The model under review builds one solid part; all positions refer to its coordinate system, in mm. Face numbers are marked on the shaded views. Round coordinates to 2 decimals unless told otherwise and drop trailing zeros. Order: outer loops, then holes, each group sorted by start corner. A loop starts at its lowest first (then second) coordinate and runs counter-clockwise, first axis right, second up.
from build123d import *

# Parameters (mm, degrees)
SKETCH1_W           = 76.2
SKETCH1_H           = 152.4
BOSS_EXTRUDE1_DEPTH = 76.2
SKETCH2_R           = 25.4
CUT_EXTRUDE1_DEPTH  = 101.6
CUT_EXTRUDE2_DEPTH  = 132.982271537
FILLET1_R           = 25.4
SKETCH4_W           = 76.2
SKETCH4_H           = 76.2
SKETCH4_R           = 12.7
CUT_EXTRUDE3_DEPTH  = 12.7
FILLET2_R           = 12.7
SKETCH6_W           = 83.912866254
SKETCH6_H           = 103.792472971
CUT_EXTRUDE4_DEPTH  = 25.4
SKETCH7_W           = 80.804571494
SKETCH7_H           = 97.595131804
CUT_EXTRUDE5_DEPTH  = 25.4


with BuildPart() as part:
    # Sketch1 → Boss-Extrude1 (new body)
    with BuildSketch(Plane.XY):
        Rectangle(SKETCH1_W, SKETCH1_H)
    extrude(amount=BOSS_EXTRUDE1_DEPTH)

    # Sketch2 → Cut-Extrude1 (cut)
    with BuildSketch(Plane(origin=(38.1, 0, 0), x_dir=(0, 0, -1), z_dir=(1, 0, 0))):
        with Locations((-38.1, 0)):
            Circle(SKETCH2_R)
    extrude(amount=-CUT_EXTRUDE1_DEPTH, mode=Mode.SUBTRACT)

    # Sketch3 → Cut-Extrude2 (cut, through all)
    with BuildSketch(Plane(origin=(38.1, 0, 0), x_dir=(0, 0, -1), z_dir=(1, 0, 0))):
        Polygon((-76.2, 0), (-50.8, -76.2), (-76.2, -76.2), align=None)
        Polygon((0, 0), (-25.4, -76.2), (0, -76.2), align=None)
    extrude(amount=-CUT_EXTRUDE2_DEPTH, mode=Mode.SUBTRACT)

    # Fillet1
    fillet1_edges = [part.edges().sort_by_distance(p)[0] for p in [
        (0, 0, 76.2),
        (0, 0, 0),
    ]]
    fillet(fillet1_edges, radius=FILLET1_R)

    # Sketch4 → Cut-Extrude3 (cut)
    with BuildSketch(Plane(origin=(0, 76.2, 0), x_dir=(1, 0, 0), z_dir=(0, 1, 0))):
        with Locations((0, -38.1)):
            Rectangle(SKETCH4_W, SKETCH4_H)
        with Locations(Location((0, -38.123369208, 0), (0, 0, 270))):
            Circle(SKETCH4_R, mode=Mode.SUBTRACT)
    extrude(amount=-CUT_EXTRUDE3_DEPTH, mode=Mode.SUBTRACT)

    # Fillet2
    fillet2_edges = [part.edges().sort_by_distance(p)[0] for p in [
        (0, 76.2, 25.423369208),
    ]]
    fillet(fillet2_edges, radius=FILLET2_R - 0.0001)  # a hair under: the kernel refuses the full size

    # Sketch6 → Cut-Extrude4 (cut)
    with BuildSketch(Plane(origin=(0, 28.172957058, 65.921201736), x_dir=(-1, 0, 0), z_dir=(0, -0.3929882709190667, -0.9195434839745439))):
        with Locations((0.104629509, -13.705043198)):
            Rectangle(SKETCH6_W, SKETCH6_H)
    extrude(amount=-CUT_EXTRUDE4_DEPTH, mode=Mode.SUBTRACT)

    # Sketch7 → Cut-Extrude5 (cut)
    with BuildSketch(Plane(origin=(0, 0.638561447, -1.491407194), x_dir=(-1, 0, 0), z_dir=(0, 0.39360002771646513, -0.9192817947624101))):
        with Locations((0.629646012, 18.826047721)):
            Rectangle(SKETCH7_W, SKETCH7_H)
    extrude(amount=CUT_EXTRUDE5_DEPTH, mode=Mode.SUBTRACT)


solid = part.part
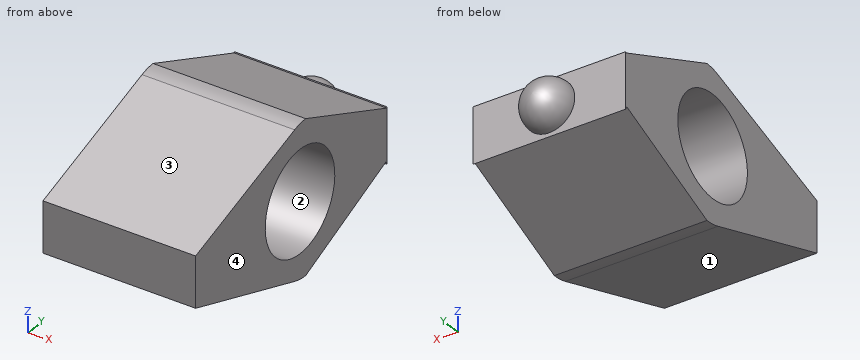
(1) Clearance check with flat-ended pins moving along their axes: P1, Ø4, axis at x = 16, y = -35.5, coming from the +Z side; P2, Ø4, axis at x = -8, y = 52.5, coming from the -Z side; P3, Ø6, axis at x = 14.5, y = -22.5, coming from the -Z side. State where each tip first meets the part, or that it passes through.
(2) To check wall thickness, follow L1, parallel to Y at x = 15, z = 38; L2, parallel to Y at x = 21, z = 45.5; L3, parallel to Z at x = 0, y = -15. State the ranges of each line that lie inside material, in increasing order.
(3) We need section A-A (x = -32). Give the boundary of the cut face in (y, z).
(4) We need section B-B (z = 57.5). Give the boundary of the cut face in (x, y).
(5) The part is to be moulded in two halves that separate along Z. For the marked faces 1, 2, 3 and 4, say which applies: pulls with the +Z half, pulls with the -Z half, needs draft (parallel to the pull), parting line crosses it, or undercut.
(6) We need section C-C (y = 0). Give the boundary of the cut face in (x, z).
(7) We need section D-D (y = -60). Give the boundary of the cut face in (x, z).
Verdict:
1. P1: stops at z = 65.03
1. P2: stops at z = 19.86
1. P3: stops at z = 6.5
2. L1: y = -76.2 to -25.4, 25.4 to 63.5
2. L2: y = -76.2 to -24.3, 24.3 to 63.5
2. L3: z = 5 to 17.6, 58.6 to 71.2
3. outline: (-76.2, 25.4) - (-3.91, 1.3) arc R25.4 ccw to (4.12, 0) - (62.8, 25.13) - (63.5, 23.5) - (63.5, 51.4) - (63.29, 50.91) - (4.12, 76.2) arc R25.4 ccw to (-3.91, 74.9) - (-76.2, 50.8) - close; hole circle Ø50.8 at (0, 38.1)
4. outline: (-38.1, -56.1) - (38.1, -56.1) - (38.1, -16.4) - (-38.1, -16.4) - close; (-38.1, 16.4) - (38.1, 16.4) - (38.1, 47.88) - (-38.1, 47.88) - close
5. face 1: pulls with the -Z half
5. face 2: undercut
5. face 3: pulls with the +Z half
5. face 4: needs draft
6. outline: (-38.1, 0.34) - (38.1, 0.34) - (38.1, 12.7) - (-38.1, 12.7) - close; (-38.1, 63.5) - (38.1, 63.5) - (38.1, 75.86) - (-38.1, 75.86) - close
7. outline: (-38.1, 20) - (38.1, 20) - (38.1, 56.2) - (-38.1, 56.2) - close
